Answer from the drawing. Dimensions are ordinates in mm from the lowest x, y and z of the part. Give positions to 0.01 mm unless a question says otherwise; leave off trailing zeros. Order: outer loops, then holes, each group sorted by start corner. A loop starts at its lowest first (then second) coordinate and runs counter-clockwise, first axis right, second up.
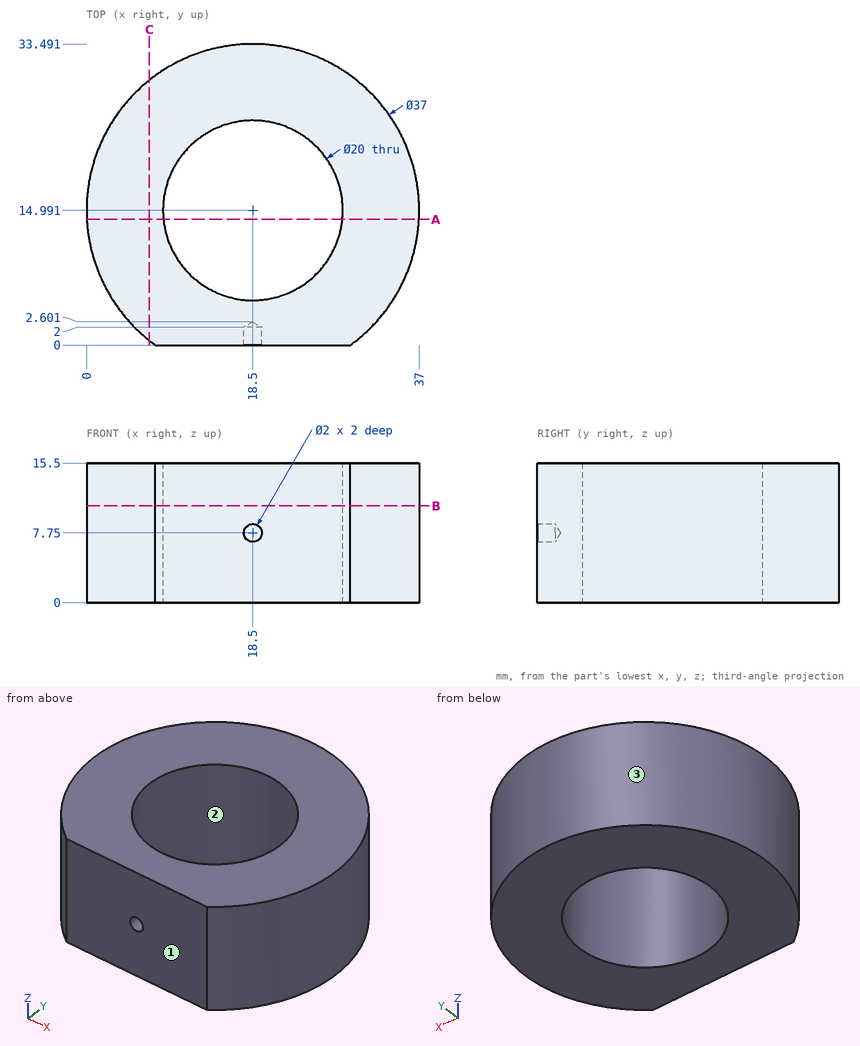
1) The part is cut by section B-B on z = 10.75. Determine the outline of the cut face in (x, y), and give its area (3 significant figures).
Final values:
outline: (7.66, 0) - (29.34, 0) arc R18.5 ccw (long way) to start; hole circle Ø20 at (18.5, 14.99)
area: 709 mm2
2) For a pull along X with two mould halves and no side action, classify the marked faces 1, 2 and 3 as released by +X, released by -X, zero draft, split by the parting line, or undercut.
Final values:
face 1: zero draft
face 2: undercut
face 3: split by the parting line
3) The part is cut by section A-A on y = 14. Determine the outline of the cut face in (x, z).
Final values:
outline: (0.03, 0) - (8.55, 0) - (8.55, 15.5) - (0.03, 15.5) - close; (28.45, 0) - (36.97, 0) - (36.97, 15.5) - (28.45, 15.5) - close
4) Given pin 1 (1 mm diameter, centred on x = 15.5, z = 7.5, fed in from +Y); pin 2 (8 mm diameter, centred on x = 10.5, z = 11, fed in from +Y); pin 3 (3 mm diameter, centred on y = 22, z = 12, fed in from -X), each flat-ended and moving along its own axis, determine where each tip first touches the part or whether it passes through.
Final values:
pin 1: stops at y = 33.32
pin 2: stops at y = 33.05
pin 3: stops at x = 0.84
5) Consider L1, parallel to X at y = 16.5, z = 12.5 (1 decimal); L2, parallel to Y at x = 25, z = 9.5; L3, parallel to X at y = 16, z = 14.75. Determine where each line is inside the solid, lowest interval first.
Final values:
L1: x = 0.1 to 8.6, 28.4 to 36.9
L2: y = 0 to 7.39, 22.59 to 32.31
L3: x = 0.03 to 8.55, 28.45 to 36.97
6) The part is cut by section C-C on x = 7. Determine the outline of the cut face in (y, z).
Final values:
outline: (0.5, 0) - (29.48, 0) - (29.48, 15.5) - (0.5, 15.5) - close
